Source: CAD feature listing. Evaluate the final solid. Frame: model axes, mm. A direction names the side the tool comes from. Give positions to 0.01 mm unless a question says otherwise; leave off trailing zeros. Write each loop counter-clockwise with the first axis right and the second up, starting at its lowest first coordinate (ties: lowest second). Pieces come first, ordered by that corner, then holes. Notation, with made-up numbers: (24.5, -37) -> (48.5, -37) arc R13 cw to (48.5, -28) -> close; hole circle Ø2 at (67.25, 37.25). An arc over 180 degrees is marked (long way). Write item = value, one per line.
from build123d import *

# Parameters (mm, degrees)
F0_W          = 10.5
F0_H          = 10.5
F1_DEPTH      = 1.5
F3_DEPTH      = 5
F5_DEPTH      = 6.75
F5_DEPTH_BACK = 6.75


# Not quite as in the source:
# - an extrude ends at something that could not be found from the text; its depth is read off the source's solid


with BuildPart() as f1:
    # F0 (on Front) → F1 (new body)
    with BuildSketch(Plane.XZ):
        Rectangle(F0_W, F0_H)
    extrude(amount=F1_DEPTH)

    # F2 (on face) → F3 (join)
    with BuildSketch(Plane(origin=(0, 0, 0), x_dir=(-1, 0, 0), z_dir=(0, 1, 0))):
        Polygon((-6.75, -5.25), (-5.25, -5.25), (-5.25, 5.25), (5.25, 5.25), (5.25, -5.25), (6.75, -5.25), (6.75, 6.75), (-6.75, 6.75), align=None)
    extrude(amount=-F3_DEPTH)

    # F4 (on Right) → F5 (join, two sides)
    with BuildSketch(Plane.YZ) as f5_sk:
        Polygon((0, 6.75), (0, -5.25), (2.8927646712, -5.25), (6.6605316242, -1.482233047), align=None)
        Polygon((2.0643375465, -3.25), (0.2965705935, -1.482233047), (2.0643375465, 0.2855339059), (3.8321044994, -1.482233047), align=None, mode=Mode.SUBTRACT)
    extrude(amount=F5_DEPTH)
    extrude(f5_sk.sketch, amount=-F5_DEPTH_BACK)


solid = f1.part
(1) Access query for faces 5 (the face through (0, 0, -5.25)), 6 (the face through (0.09, 1.17, -0.61)), 7 (the face through (5.25, -3, 0)). Directions: +Z, -Z, +X, -X, +Y, -Y. A direction counts if a zero-diameter tool reaches every point of the face in a straight line with its end or side. Return the directions, or none.
Values follow:
face_5 = -Z, +X, -X, +Y, -Y
face_6 = +X, -X
face_7 = -Z, -Y
(2) First-contact query: pin 1 (5 mm diameter, centred on x = -4, z = 2, fed in from +Y); pin 2 (1.5 mm diameter, centred on x = -1.5, z = -3.5, fed in from -Y); pin 3 (5 mm diameter, centred on x = 4.5, z = 1.5, fed in from +Y). Flat tips, straight axial feed; report the tip coordinate or a pass-through.
Values follow:
pin_1 = 5.87
pin_2 = -1.5
pin_3 = 6.27
(3) Material intervals for line 1 (X direction, y = -2, z = -1); line 2 (Z direction, x = 3.75, y = -3); line 3 (Z direction, x = -5.5, y = 2.25), sorted ascending.
Values follow:
line_1 = -6.75 to -5.25, 5.25 to 6.75
line_2 = 5.25 to 6.75
line_3 = -5.25 to -3.06, 0.1 to 3.97
(4) Section query B-B (y = 0.5). Return loops of the section in (x, z), plus the area to 3 significant figures.
Values follow:
outline = (-6.75, -5.25) -> (6.75, -5.25) -> (6.75, -1.69) -> (-6.75, -1.69) -> close; (-6.75, -1.28) -> (6.75, -1.28) -> (6.75, 6.13) -> (-6.75, 6.13) -> close
area = 148 mm2
(5) Pull-direction query (Z, two-part tool) for faces 1 (the face through (0.09, 4.75, -3.39)), 2 (the face through (0.095, 1.193, -2.378)), 3 (the face through (0.095, 2.961, -2.354)), 4 (the face through (0.095, 3.377, 2.576)); classes: pulls with the +Z half, pulls with the -Z half, needs draft (parallel to the pull), parting line crosses it, or undercut.
Values follow:
face_1 = pulls with the -Z half
face_2 = undercut
face_3 = undercut
face_4 = pulls with the +Z half
(6) Section query A-A (x = -1.5). Return loops of the section in (y, z), plus the area to 3 significant figures.
Values follow:
outline = (-5, 5.25) -> (-1.5, 5.25) -> (-1.5, -5.25) -> (2.89, -5.25) -> (6.66, -1.48) -> (0, 6.75) -> (-5, 6.75) -> close; hole (0.3, -1.48) -> (2.06, -3.25) -> (3.83, -1.48) -> (2.06, 0.29) -> close
area = 62.4 mm2
(7) Section query D-D (x = -6). Return loops of the section in (y, z), plus the area to 3 significant figures.
Values follow:
outline = (-5, -5.25) -> (2.89, -5.25) -> (6.66, -1.48) -> (0, 6.75) -> (-5, 6.75) -> close; hole (0.3, -1.48) -> (2.06, -3.25) -> (3.83, -1.48) -> (2.06, 0.29) -> close
area = 99.2 mm2
(8) Section query C-C (y = -2.25). Return loops of the section in (x, z), plus the area to 4 significant figures.
Values follow:
outline = (-6.75, -5.25) -> (-5.25, -5.25) -> (-5.25, 5.25) -> (5.25, 5.25) -> (5.25, -5.25) -> (6.75, -5.25) -> (6.75, 6.75) -> (-6.75, 6.75) -> close
area = 51.75 mm2
